```python
from build123d import *

# Parameters (mm, degrees)
ESQUISSE1_R             = 2.5
BASE_EXTRUSION_DEPTH    = 228
CHANFREIN1_SIZE         = 0.5
ESQUISSE2_R             = 1
ENL_V_MAT_EXTRU_1_DEPTH = 50


with BuildPart() as part:
    # Esquisse1 → Base-Extrusion (new body)
    with BuildSketch(Plane.XY):
        Circle(ESQUISSE1_R)
    extrude(amount=BASE_EXTRUSION_DEPTH)

    # Chanfrein1
    chanfrein1_edges = [part.edges().sort_by_distance(p)[0] for p in [
        (-2.5, 0, 0),
        (-2.5, 0, 228),
    ]]
    chamfer(chanfrein1_edges, length=CHANFREIN1_SIZE)

    # Esquisse2 → Enlèv. mat.-Extru.1 (cut, symmetric)
    with BuildSketch(Plane(origin=(0, 0, 0), x_dir=(1, 0, 0), z_dir=(0, 1, 0))):
        with Locations((0, -17)):
            Circle(ESQUISSE2_R)
        with Locations((0, -211)):
            Circle(ESQUISSE2_R)
    extrude(amount=ENL_V_MAT_EXTRU_1_DEPTH, both=True, mode=Mode.SUBTRACT)


solid = part.part
```
Source: CAD feature listing. Evaluate the final solid. Frame: model axes, mm. Coordinates: 2 decimals unless noted, no trailing zeros. Write each loop counter-clockwise with the first axis right and the second up, starting at its lowest first coordinate (ties: lowest second). Pieces come first, ordered by that corner, then holes. Notation, with made-up numbers: (72, -23) - (105, -23) arc R21 ccw to (105, 7) - close; hole circle Ø7 at (83.5, 29.25). An arc over 180 degrees is marked (long way). Answer as a JSON object with one key per item and string values.
Q1. Material intervals for line 1 (Z direction, x = 0, y = 1.45); line 2 (X direction, y = 0.3, z = 211); line 3 (X direction, y = -0.4, z = 161), sorted ascending. Write a range as [from, to].
Ans:
{"line 1": "z = [0, 16], [18, 210], [212, 228]", "line 2": "x = [-2.48, -1], [1, 2.48]", "line 3": "x = [-2.47, 2.47]"}
Q2. Section query A-A, the plane x = 0. Output: boundary loops of the cut face in (y, z).
Ans:
{"outline": "(-2.5, 0.5) - (-2, 0) - (2, 0) - (2.5, 0.5) - (2.5, 16) - (-2.5, 16) - close; (-2.5, 18) - (2.5, 18) - (2.5, 210) - (-2.5, 210) - close; (-2.5, 212) - (2.5, 212) - (2.5, 227.5) - (2, 228) - (-2, 228) - (-2.5, 227.5) - close"}
Q3. Section query B-B, the plane z = 192. Output: boundary loops of the cut face in (x, y), plus the area to 3 significant figures.
Ans:
{"outline": "circle Ø5 at (0, 0)", "area": "19.6 mm2"}
Q4. First-contact query: pin 1 Ø1.6 at (x, z) = (0, 211) entering from -Y; pin 2 Ø2 at (x, z) = (2, 50.5) entering from -Y. Flat tips, straight axial feed; report the tip coordinate or a pass-through.
Ans:
{"pin 1": "passes through", "pin 2": "stops at y = -2.29"}
Q5. Section query C-C, the plane y = -0.8. State how many separate pieces and enclosed holes the cut face has, plus the area to 3 significant figures.
Ans:
{"separate pieces": "1", "enclosed holes": "2", "area": "1,070 mm2"}
